Autodesk Inventor part; units mm, degrees
ref_plane "YZ Plane" through (0, 0, 0) normal (1, 0, 0) x (0, 1, 0)
ref_plane "XZ Plane" through (0, 0, 0) normal (0, 1, 0) x (-1, 0, 0)
ref_plane "XY Plane" through (0, 0, 0) normal (0, 0, 1) x (1, 0, 0)
sketch "Sketch1" plane through (0, 0, 0) normal (0, 0, 1) x (1, 0, 0)
  line L0 (0, 0) -> (127, 0)
  line L1 (127, 0) -> (127, 76.2)
  line L2 (127, 76.2) -> (0, 76.2)
  line L3 (0, 76.2) -> (0, 0)
  circle A0 centre (63.5, 38.1) radius 9.525
  circle A1 centre (63.5, 63.5) radius 2.0193
  circle A2 centre (38.1, 38.1) radius 2.0193
  circle A3 centre (63.5, 12.7) radius 2.0193
  circle A4 centre (88.9, 38.1) radius 2.0193
  circle A5 centre (12.7, 63.5) radius 3.2512
  circle A6 centre (12.7, 38.1) radius 3.2512
  circle A7 centre (12.7, 12.7) radius 3.2512
  circle A8 centre (114.3, 63.5) radius 3.2512
  circle A9 centre (114.3, 38.1) radius 3.2512
  circle A10 centre (114.3, 12.7) radius 3.2512
  dimension "d0" = 127
  dimension "d1" = 76.2
  dimension "d2" = 19.05
  dimension "d3" = 38.1
  dimension "d4" = 63.5
  dimension "d5" = 4.0386
  dimension "d6" = 25.4
  dimension "d7" = 63.5
  dimension "d8" = 4.0386
  dimension "d9" = 25.4
  dimension "d10" = 38.1
  dimension "d13" = 50.8
  dimension "d20" = 50.8
  dimension "d25" = 6.5024
  dimension "d26" = 12.7
  dimension "d27" = 12.7
  dimension "d30" = 25.4
  dimension "d39" = 101.6
extrude "Extrusion2" add sketch "Sketch1" along normal blind 5.08
equation "\"d3\" = 0.5 * d1"
equation "\"d7\" = d4"
equation "\"d8\" = d5"
equation "\"d9\" = d6"
equation "\"d10\" = 0.5 * d1"
properties part number "Motor Mount Short"
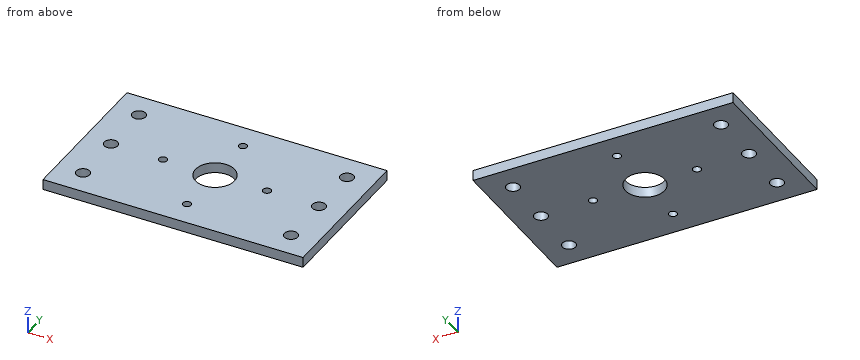
Check sheet for the modelled part. Datum: model origin and axes. Units: mm. Round coordinates to 2 decimals unless told otherwise and drop trailing zeros. Order: outer loops, then holes, each group sorted by start corner. A loop starts at its lowest first (then second) coordinate and runs counter-clockwise, first axis right, second up.
(1) Cross-section at B-B, the plane x = 63.5. Enter the section's corners in (y, z) (3 decimals), and give its area (3 significant figures).
(2) Scan lines: probe 1 along X at (y, z) = (12.5, 4.5); probe 2 along Y at (x, z) = (114.3, 3.4); probe 3 along Y at (x, z) = (13, 4.8). Record each from-to range of solid material in increasing order.
(3) Cross-section at A-A, the plane y = 38.1. Enter the section's corners in (x, z) (3 decimals), and give its area (3 significant figures).
(4) Cross-section at D-D, the plane y = 12.7. Enter the section's corners in (x, z).
(5) Cross-section at C-C, the plane z = 3.65. State how many separate pieces and enclosed holes the cut face has, and give its area (3 significant figures).
(6) Go/stop test with a flat-tipped pin: P1, Ø3.5, axis at x = 38.1, y = 38.1, coming from the +Z side. Record where the tip stops, or that it passes through.
Check sheet entries:
1. outline: (0, 0) - (10.681, 0) - (10.681, 5.08) - (0, 5.08) - close; (14.719, 0) - (28.575, 0) - (28.575, 5.08) - (14.719, 5.08) - close; (47.625, 0) - (61.481, 0) - (61.481, 5.08) - (47.625, 5.08) - close; (65.519, 0) - (76.2, 0) - (76.2, 5.08) - (65.519, 5.08) - close
1. area: 249 mm2
2. probe 1: x = 0 to 9.45, 15.95 to 61.49, 65.51 to 111.05, 117.55 to 127
2. probe 2: y = 0 to 9.45, 15.95 to 34.85, 41.35 to 60.25, 66.75 to 76.2
2. probe 3: y = 0 to 9.46, 15.94 to 34.86, 41.34 to 60.26, 66.74 to 76.2
3. outline: (0, 0) - (9.449, 0) - (9.449, 5.08) - (0, 5.08) - close; (15.951, 0) - (36.081, 0) - (36.081, 5.08) - (15.951, 5.08) - close; (40.119, 0) - (53.975, 0) - (53.975, 5.08) - (40.119, 5.08) - close; (73.025, 0) - (86.881, 0) - (86.881, 5.08) - (73.025, 5.08) - close; (90.919, 0) - (111.049, 0) - (111.049, 5.08) - (90.919, 5.08) - close; (117.551, 0) - (127, 0) - (127, 5.08) - (117.551, 5.08) - close
3. area: 441 mm2
4. outline: (0, 0) - (9.45, 0) - (9.45, 5.08) - (0, 5.08) - close; (15.95, 0) - (61.48, 0) - (61.48, 5.08) - (15.95, 5.08) - close; (65.52, 0) - (111.05, 0) - (111.05, 5.08) - (65.52, 5.08) - close; (117.55, 0) - (127, 0) - (127, 5.08) - (117.55, 5.08) - close
5. separate pieces: 1
5. enclosed holes: 11
5. area: 9,140 mm2
6. P1: passes through
